```python
from build123d import *

# Parameters (mm, degrees)
SKETCH_R          = 1.6
PAD_DEPTH         = 6
SKETCH001_R       = 3
POCKET_DEPTH      = 40.001
POCKET_DEPTH_BACK = -40.001


with BuildPart() as toolbody:
    # Sketch → Pad (new body)
    with BuildSketch(Plane.XY):
        Polygon((0, 40), (46, 40), (56, 40), (56, -40), (46, -40), (0, -40), (0, -25), (17.5, -25), (0, -7.5), (0, 7.5), (17.5, 25), (0, 25), align=None)
        with Locations((53, 0)):
            Circle(SKETCH_R, mode=Mode.SUBTRACT)
        with Locations((53, 35)):
            Circle(SKETCH_R, mode=Mode.SUBTRACT)
        with Locations((53, -35)):
            Circle(SKETCH_R, mode=Mode.SUBTRACT)
        with Locations((39, 35)):
            Circle(SKETCH_R, mode=Mode.SUBTRACT)
        with Locations((39, 0)):
            Circle(SKETCH_R, mode=Mode.SUBTRACT)
        with Locations((39, -35)):
            Circle(SKETCH_R, mode=Mode.SUBTRACT)
        with Locations((15, 35)):
            Circle(SKETCH_R, mode=Mode.SUBTRACT)
        with Locations((15, -35)):
            Circle(SKETCH_R, mode=Mode.SUBTRACT)
        Polygon((15, 0), (28.75, 13.75), (28.75, -13.75), align=None, mode=Mode.SUBTRACT)
    extrude(amount=-PAD_DEPTH)

    # Sketch001 → Pocket (cut, two sides)
    with BuildSketch(Plane.XZ) as pocket_sk:
        with Locations((46, 0)):
            Circle(SKETCH001_R)
    extrude(amount=-POCKET_DEPTH, mode=Mode.SUBTRACT)
    extrude(pocket_sk.sketch, amount=-POCKET_DEPTH_BACK, mode=Mode.SUBTRACT)


with BuildPart() as toolfusion:
    # Part__Mirroring: instance of ToolBody
    add(toolbody.part.mirror(Plane(origin=(0, 0, 0), x_dir=(0, -1, 0), z_dir=(1, 0, 0))))

    # Fusion: union ToolBody
    add(toolbody.part)


solid = toolfusion.part
```
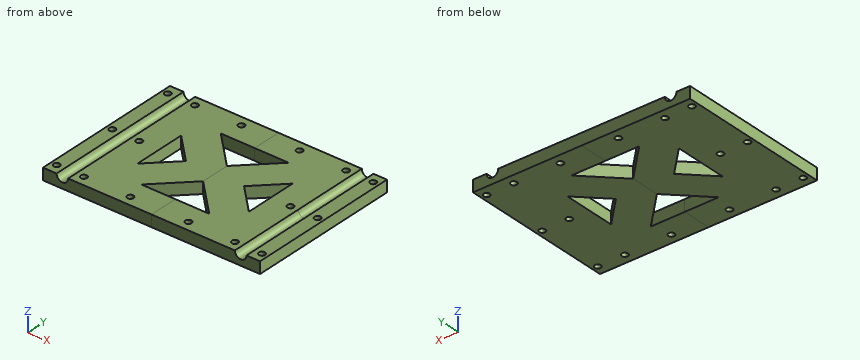
For this review, take the finished solid that the model builds, in its own axes (mm). Give positions to 0.01 mm unless a question says otherwise; leave off trailing zeros. Write each loop counter-clockwise with the first axis right and the second up, starting at its lowest first coordinate (ties: lowest second). Pieces come first, ordered by that corner, then holes. Notation, with made-up numbers: M 37,18 L 57,18 A10 ccw 57,31 Z; hole C 1,43.25 d11. An arc over 180 degrees is marked long. One line per item, written item: value.
1) Take a section at B-B, the plane y = 35. Count the separate pieces of the cut face and the enclosed holes in it, then the cut area to 3 significant figures.
Results are:
separate pieces: 7
enclosed holes: 0
area: 529 mm²
2) Take a section at A-A, the plane x = -5. Write out the cut boundary in (y, z).
Results are:
outline: M -40,-6 L -25,-6 L -25,0 L -40,0 Z; M -12.5,-6 L 12.5,-6 L 12.5,0 L -12.5,0 Z; M 25,-6 L 40,-6 L 40,0 L 25,0 Z
3) Take a section at C-C, the plane x = -19.5. Write out the cut boundary in (y, z), then the cut area to 3 significant figures.
Results are:
outline: M -40,-6 L -4.5,-6 L -4.5,0 L -40,0 Z; M 4.5,-6 L 40,-6 L 40,0 L 4.5,0 Z
area: 426 mm²
4) For P1, Ø3.5, axis at x = 15, y = -35, coming from the -Z side, flat-tipped, find the tip position at first contact; note if it passes through.
Results are:
P1: stops at z = -6
5) For line 1 (Y direction, x = 39, z = -1.5); line 2 (X direction, y = 15, z = -0.3); line 3 (X direction, y = -16, z = -2.25), list the stretches that pass through material, from the lowest coordinate up. Write a range as from..to.
Results are:
line 1: y = -40..-36.6, -33.4..-1.6, 1.6..33.4, 36.6..40
line 2: x = -56..-48.98, -43.02..-7.5, 7.5..43.02, 48.98..56
line 3: x = -56..-47.98, -44.02..-8.5, 8.5..44.02, 47.98..56
